```python
from build123d import *

# Parameters (mm, degrees)
SKETCH1_W           = 31
SKETCH1_H           = 16
BOSS_EXTRUDE1_DEPTH = 58
SKETCH2_W           = 17
SKETCH2_H           = 21
BOSS_EXTRUDE2_DEPTH = 58
SKETCH3_W           = 10
SKETCH3_H           = 6
BOSS_EXTRUDE3_DEPTH = 58
CHAMFER1_SIZE       = 1
CHAMFER2_SIZE       = 1.5
CHAMFER5_SIZE2      = 3.501037691
CHAMFER5_SIZE       = 5
CHAMFER6_SIZE2      = 5
CHAMFER6_SIZE       = 3.501037691
SKETCH4_R           = 7.5
CUT_EXTRUDE1_DEPTH  = 1
CUT_EXTRUDE2_START  = -1
SKETCH5_R           = 7.5
CUT_EXTRUDE2_DEPTH  = 1
SKETCH6_R           = 4
CUT_EXTRUDE3_DEPTH  = 58
SKETCH7_R           = 2
CUT_EXTRUDE4_DEPTH  = 20
SKETCH8_R           = 6.75
SKETCH8_R_2         = 4.75
CUT_EXTRUDE5_DEPTH  = 0.1
CUT_EXTRUDE6_START  = -0.1
SKETCH9_R           = 6.75
SKETCH9_R_2         = 4.75
CUT_EXTRUDE6_DEPTH  = 0.1
FILLET1_R           = 0.5
FILLET2_START       = -1
FILLET2_DEPTH       = 60


with BuildPart() as part:
    # Sketch1 → Boss-Extrude1 (new body)
    with BuildSketch(Plane.XY):
        Rectangle(SKETCH1_W, SKETCH1_H)
    extrude(amount=BOSS_EXTRUDE1_DEPTH)

    # Sketch2 → Boss-Extrude2 (add)
    with BuildSketch(Plane.XY.offset(58)):
        with Locations((0, -2.5)):
            Rectangle(SKETCH2_W, SKETCH2_H)
    extrude(amount=-BOSS_EXTRUDE2_DEPTH)

    # Sketch3 → Boss-Extrude3 (add)
    with BuildSketch(Plane.XY.offset(58)):
        with Locations((-12, 6)):
            Rectangle(SKETCH3_W, SKETCH3_H)
        with Locations((12, 6)):
            Rectangle(SKETCH3_W, SKETCH3_H)
    extrude(amount=-BOSS_EXTRUDE3_DEPTH)

    # Chamfer1
    chamfer1_edges = [part.edges().sort_by_distance(p)[0] for p in [
        (7, 8, 29),
        (-7, 8, 29),
    ]]
    chamfer(chamfer1_edges, length=CHAMFER1_SIZE - 0.0001)  # a hair under: the kernel refuses the full size

    # Chamfer2
    chamfer2_edges = [part.edges().sort_by_distance(p)[0] for p in [
        (15.5, 3, 29),
        (-15.5, 3, 29),
    ]]
    chamfer(chamfer2_edges, length=CHAMFER2_SIZE - 0.0001)  # a hair under: the kernel refuses the full size

    # Chamfer5
    chamfer5_edges = [part.edges().sort_by_distance(p)[0] for p in [
        (-8.5, -13, 29),
    ]]
    chamfer5_side = [part.faces().sort_by_distance(p)[0] for p in [
        (-8.5, -12.929979246, 29),
    ]]
    chamfer(chamfer5_edges, length=CHAMFER5_SIZE - 0.0001, length2=CHAMFER5_SIZE2 - 0.0001, reference=chamfer5_side[0])  # a hair under: the kernel refuses the full size

    # Chamfer6
    chamfer6_edges = [part.edges().sort_by_distance(p)[0] for p in [
        (8.5, -13, 29),
    ]]
    chamfer6_side = [part.faces().sort_by_distance(p)[0] for p in [
        (8.429979246, -13, 29),
    ]]
    chamfer(chamfer6_edges, length=CHAMFER6_SIZE - 0.0001, length2=CHAMFER6_SIZE2 - 0.0001, reference=chamfer6_side[0])  # a hair under: the kernel refuses the full size

    # Sketch4 → Cut-Extrude1 (cut)
    with BuildSketch(Plane.XY.offset(58)):
        with Locations((0, -2)):
            Circle(SKETCH4_R)
    extrude(amount=-CUT_EXTRUDE1_DEPTH, mode=Mode.SUBTRACT)

    # Sketch5 → Cut-Extrude2 (cut)
    with BuildSketch(Plane(origin=(0, 0, 0), x_dir=(-1, 0, 0), z_dir=(0, 0, -1)).offset(CUT_EXTRUDE2_START)):
        with Locations(Location((0, -2, 0), (0, 0, 180))):
            Circle(SKETCH5_R)
    extrude(amount=CUT_EXTRUDE2_DEPTH, mode=Mode.SUBTRACT)

    # Sketch6 → Cut-Extrude3 (cut)
    with BuildSketch(Plane(origin=(0, 0, 1), x_dir=(-1, 0, 0), z_dir=(0, 0, -1))):
        with Locations((0, -2)):
            Circle(SKETCH6_R)
    extrude(amount=-CUT_EXTRUDE3_DEPTH, mode=Mode.SUBTRACT)

    # Sketch7 → Cut-Extrude4 (cut)
    with BuildSketch(Plane(origin=(0, 9, 0), x_dir=(1, 0, 0), z_dir=(0, 1, 0))):
        with Locations(Location((-12, -8, 0), (0, 0, 180))):
            Circle(SKETCH7_R)
        with Locations(Location((12, -8, 0), (0, 0, 180))):
            Circle(SKETCH7_R)
        with Locations(Location((12, -50, 0), (0, 0, 180))):
            Circle(SKETCH7_R)
        with Locations(Location((-12, -50, 0), (0, 0, 180))):
            Circle(SKETCH7_R)
    extrude(amount=-CUT_EXTRUDE4_DEPTH, mode=Mode.SUBTRACT)

    # Sketch8 → Cut-Extrude5 (cut)
    with BuildSketch(Plane.XY.offset(57)):
        with Locations((0, -2)):
            Circle(SKETCH8_R)
        with Locations((0, -2)):
            Circle(SKETCH8_R_2, mode=Mode.SUBTRACT)
    extrude(amount=-CUT_EXTRUDE5_DEPTH, mode=Mode.SUBTRACT)

    # Sketch9 → Cut-Extrude6 (cut)
    with BuildSketch(Plane(origin=(0, 0, 1), x_dir=(-1, 0, 0), z_dir=(0, 0, -1)).offset(CUT_EXTRUDE6_START)):
        with Locations(Location((0, -2, 0), (0, 0, 180))):
            Circle(SKETCH9_R)
        with Locations(Location((0, -2, 0), (0, 0, 180))):
            Circle(SKETCH9_R_2, mode=Mode.SUBTRACT)
    extrude(amount=CUT_EXTRUDE6_DEPTH, mode=Mode.SUBTRACT)

    # Fillet1
    fillet1_edges = [part.edges().sort_by_distance(p)[0] for p in [
        (-4.999062309, -13, 29),
        (4.999062309, -13, 29),
        (-17, 9, 29),
        (17, 9, 29),
        (15.5, -8, 29),
        (-15.5, -8, 29),
    ]]
    fillet(fillet1_edges, radius=FILLET1_R)

    # Fillet2: read off the stored shape, not the designer's step
    # Fillet2 outline → Fillet2 (cut)
    with BuildSketch(Plane.XY.offset(FILLET2_START)):
        with BuildLine():
            Line((7, 9), (6.853553391, 8.853553391))
            ThreePointArc((6.853553391, 8.853553391), (7.015765065, 8.961939766), (7.207106781, 9))
            Line((7.207106781, 9), (7, 9))
        make_face()
        with BuildLine():
            Line((-7, 9), (-7.207106781, 9))
            ThreePointArc((-7.207106781, 9), (-7.015765065, 8.961939766), (-6.853553391, 8.853553391))
            Line((-6.853553391, 8.853553391), (-7, 9))
        make_face()
    extrude(amount=FILLET2_DEPTH, mode=Mode.SUBTRACT)


solid = part.part
```
Input: part model. Units: mm. Frame: model coordinates. A direction names the side the tool comes from. Coordinates: 2 decimals unless noted, no trailing zeros. Loops run counter-clockwise (first coordinate to the right, second up) from the corner with the lowest first, then second, coordinate; pieces in that order, holes last.
Q1. Section A-A, the plane x = 12. Return the cut outline in (y, z), and give its area (3 significant figures).
Results are:
outline: (-8, 0) - (9, 0) - (9, 6) - (-8, 6) - close; (-8, 10) - (9, 10) - (9, 48) - (-8, 48) - close; (-8, 52) - (9, 52) - (9, 58) - (-8, 58) - close
area: 850 mm2
Q2. Line query: line 1 along Z through (x, y) = (12, -2); line 2 along X through (y, z) = (-2.25, 6.5); line 3 along X through (y, z) = (-4, 50.5). Output: solid intervals per line, ascending.
Results are:
line 1: z = 0 to 6, 10 to 48, 52 to 58
line 2: x = -15.5 to -13.32, -10.68 to -3.99, 3.99 to 10.68, 13.32 to 15.5
line 3: x = -15.5 to -13.94, -10.06 to -3.46, 3.46 to 10.06, 13.94 to 15.5
Q3. Contact query for flat-ended pins moving along their axis: pin 1 (7 mm diameter, centred on x = 12.5, z = 27.5, fed in from -Y); pin 2 (4 mm diameter, centred on x = 1, y = 0.5, fed in from +Z); pin 3 (8 mm diameter, centred on y = -4.5, z = 35, fed in from +X); pin 4 (2.5 mm diameter, centred on x = -12, z = 8, fed in from -Y). Output: stop coordinate, or through.
Results are:
pin 1: stops at y = -8
pin 2: stops at z = 57
pin 3: stops at x = 15.5
pin 4: passes through
Q4. Section D-D, the plane y = -2. Give the number of separate pieces and of enclosed holes in the cut face, and give its area (3 significant figures).
Results are:
separate pieces: 2
enclosed holes: 4
area: 1,270 mm2
Q5. Set-up query: faces 5 (the flat face through (1, 3, 56.9)), 6 (the flat face through (-12, -8, 29)), 7 (the flat face through (12, -8, 29)), 8 (the flat face through (-5, -1, 1.1)), 9 (the flat face through (0, 8, 29)). Return all of +Z, -Z, +X, -X, +Y, -Y with unobstructed straight access to the full face (end or side cutting, diameter ignored); none if empty.
Results are:
face 5: +Z
face 6: +Z, -Z, -X, -Y
face 7: +Z, -Z, +X, -Y
face 8: -Z
face 9: +Z, -Z, +Y
Q6. Mould query, pull axis X, two halves, no side actions, for faces 1 (the cylindrical face through (-3.815, -0.799, 28.608)), 2 (the flat face through (-6.8, -10.43, 29.41)), 3 (the flat face through (4, 5, 58)), 4 (the flat face through (17, 6, 29)). Classes: +X half, -X half, draft (parallel to the pull), parting line (faces both ways), or undercut.
Results are:
face 1: undercut
face 2: -X half
face 3: draft
face 4: +X half
